```python
from build123d import *

# Parameters (mm, degrees)
SKETCH_1_W      = 40
SKETCH_1_H      = 20
EXTRUDE_1_DEPTH = 40
EXTRUDE_START   = -27.5
EXTRUDE_4_DEPTH = 3
SKETCH_2_R      = 3
EXTRUDE_5_DEPTH = 6
SKETCH_8_W      = 34
SKETCH_8_H      = 15
EXTRUDE_6_DEPTH = 1.5
FILLET_1_R      = 1.5
SKETCH_9_R      = 5.130323695
EXTRUDE_7_DEPTH = 0.6
FILLET_2_R      = 1
CHAMFER_1_SIZE  = 1


# Some blends are built 0.0001 mm under size
with BuildPart() as part:
    # 草图1 → 凸台-拉伸1 (new body)
    with BuildSketch(Plane(origin=(0, 0, 0), x_dir=(1, 0, 0), z_dir=(0, 1, 0))):
        with Locations((20, -10)):
            Rectangle(SKETCH_1_W, SKETCH_1_H)
    extrude(amount=EXTRUDE_1_DEPTH)

    # 草图7 → 凸台-拉伸4 (add)
    with BuildSketch(Plane.XZ.offset(EXTRUDE_START)):
        with BuildLine():
            Line((40, 20), (47, 20))
            Line((47, 20), (47, 16.089724736))
            ThreePointArc((47, 16.089724736), (42.25, 15), (47, 13.910275264))
            Line((47, 13.910275264), (47, 6.089724736))
            ThreePointArc((47, 6.089724736), (42.25, 5), (47, 3.910275264))
            Line((47, 3.910275264), (47, 0))
            Line((47, 0), (40, 0))
            Line((40, 0), (40, 20))
        make_face()
        with BuildLine():
            Line((0, 20), (0, 0))
            Line((0, 0), (-7, 0))
            Line((-7, 0), (-7, 3.910275264))
            ThreePointArc((-7, 3.910275264), (-2.25, 5), (-7, 6.089724736))
            Line((-7, 6.089724736), (-7, 13.910275264))
            ThreePointArc((-7, 13.910275264), (-2.25, 15), (-7, 16.089724736))
            Line((-7, 16.089724736), (-7, 20))
            Line((-7, 20), (0, 20))
        make_face()
    extrude(amount=-EXTRUDE_4_DEPTH)

    # 草图2 → 凸台-拉伸5 (add)
    with BuildSketch(Plane(origin=(0, 40, 0), x_dir=(1, 0, 0), z_dir=(0, 1, 0))):
        with Locations(Location((29.9, -10, 0), (0, 0, 270))):
            Circle(SKETCH_2_R)
    extrude(amount=EXTRUDE_5_DEPTH)

    # 草图8 → 凸台-拉伸6 (add)
    with BuildSketch(Plane(origin=(0, 40, 0), x_dir=(1, 0, 0), z_dir=(0, 1, 0))):
        with Locations((20, -10.251596062)):
            Rectangle(SKETCH_8_W, SKETCH_8_H)
    extrude(amount=EXTRUDE_6_DEPTH)

    # 圆角1
    fillet_1_edges = [part.edges().sort_by_distance(p)[0] for p in [
        (20, 41.5, 2.751596062),
        (37, 41.5, 10.251596062),
        (20, 41.5, 17.751596062),
        (3, 41.5, 10.251596062),
    ]]
    fillet(fillet_1_edges, radius=FILLET_1_R - 0.0001)  # a hair under: the kernel refuses the full size

    # 草图9 → 凸台-拉伸7 (add)
    with BuildSketch(Plane(origin=(0, 41.5, 0), x_dir=(1, 0, 0), z_dir=(0, 1, 0))):
        with Locations(Location((29.9, -10, 0), (0, 0, 90))):
            Circle(SKETCH_9_R)
    extrude(amount=EXTRUDE_7_DEPTH)

    # 圆角2
    # the kernel refuses this fillet: 1 mm, written as the material it takes off along each edge
    with BuildSketch(Plane(origin=(29.9, 42.1, 10), x_dir=(0, 0, -1), z_dir=(1, 0, 0))) as fillet_2_piece_1:
        with BuildLine():
            CenterArc((4.213808556, -1), FILLET_2_R, 23.578178478, 66.421821522)
            Line((4.213808556, 0), (4.213808556, 0.02))
            Line((4.213808556, 0.02), (5.130323695, 0.02))
            Line((5.130323695, 0.02), (5.150323695, 0))
            ThreePointArc((5.150323695, 0), (5.150323695, -0.3), (5.148653998, -0.592))
            Line((5.148653998, -0.592), (5.130323695, -0.6))
        make_face()
    revolve(axis=Axis((29.9, 42.1, 10), (0, 1, 0)), mode=Mode.SUBTRACT)

    # 倒角1
    chamfer_1_edges = [part.edges().sort_by_distance(p)[0] for p in [
        (40, 40, 10),
        (20, 40, 0),
        (0, 40, 10),
        (20, 40, 20),
    ]]
    chamfer(chamfer_1_edges, length=CHAMFER_1_SIZE)


solid = part.part
```
Geometry check sheet. Reference: the model listing, model coordinates, mm. A direction names the side the tool comes from. Round coordinates to 2 decimals unless told otherwise and drop trailing zeros. Order: outer loops, then holes, each group sorted by start corner. A loop starts at its lowest first (then second) coordinate and runs counter-clockwise, first axis right, second up. Notation, with made-up numbers: M 61.25,29 L 88.25,29 A34 ccw 88.25,64 Z; hole C 27,-13.5 d4. An arc over 180 degrees is marked long. Answer as CSV lines item,"result".
1) Tool access check on faces 1 (the face through (43, 30.5, 10)), 2 (the face through (43, 27.5, 10)), 3 (the face through (18.5, 40, 2.6)), 4 (the face through (-3, 30.5, 10)). Record the directions out of +Z, -Z, +X, -X, +Y, -Y that give a thin tool (end or side, any length) a straight path to the whole face; none if there is none.
Entries:
face 1,"+Z, -Z, +X, +Y"
face 2,"+Z, -Z, +X, -Y"
face 3,"+Y"
face 4,"+Z, -Z, -X, +Y"
2) Sectioned sample at A-A on x = 44.75. Record the cut outline in (y, z), and give its area (3 significant figures).
Entries:
outline,"M 27.5,0 L 30.5,0 L 30.5,2.5 L 27.5,2.5 Z; M 27.5,7.5 L 30.5,7.5 L 30.5,12.5 L 27.5,12.5 Z; M 27.5,17.5 L 30.5,17.5 L 30.5,20 L 27.5,20 Z"
area,"30.0 mm2"
3) Sectioned sample at D-D on y = 7. Record the cut outline in (x, z).
Entries:
outline,"M 0,0 L 40,0 L 40,20 L 0,20 Z"
4) Gauge pin test, flat ends, axial feed: pin 1 Ø8 at (x, z) = (-4.75, 5) entering from +Y; pin 2 Ø4 at (y, z) = (34.5, 9.5) entering from -X; pin 3 Ø5 at (x, z) = (22, 2) entering from +Y; pin 4 Ø3 at (x, z) = (44.75, 5) entering from +Y. Record the tip position at first contact, or that the pin passes through.
Entries:
pin 1,"y = 30.5"
pin 2,"x = 0"
pin 3,"y = 41.5"
pin 4,"through"
5) Mould release check, pull along Z, two halves, no side actions. Record for faces 5 (the face through (-2.25, 28.98, 14.91)), 6 (the face through (20.238, 41.049, 17.324)), 7 (the face through (36.55, 41.07, 10.15)): +Z half, -Z half, draft (parallel to the pull), parting line (faces both ways), or undercut.
Entries:
face 5,"undercut"
face 6,"+Z half"
face 7,"draft"
6) Thickness scan on probe 1 along Z at (x, y) = (44.75, 29.35); probe 2 along Z at (x, y) = (-4, 28); probe 3 along X at (y, z) = (18.5, 14). Record the ranges inside material, lowest first. Write a range as [from, to].
Entries:
probe 1,"[0, 2.5], [7.5, 12.5], [17.5, 20]"
probe 2,"[0, 2.62], [7.38, 12.62], [17.38, 20]"
probe 3,"[0, 40]"
